Build history of the part. All positions in model axes, mm. A direction names the side the tool comes from. Round coordinates to 2 decimals unless told otherwise and drop trailing zeros. Write each loop counter-clockwise with the first axis right and the second up, starting at its lowest first coordinate (ties: lowest second). Pieces come first, ordered by that corner, then holes. Notation, with made-up numbers: (-16.5, 47.5) - (-7.5, 47.5) arc R19 cw to (-7.5, 70.5) - close; hole circle Ø7 at (-11.75, 17.5). An arc over 180 degrees is marked (long way). One line per question, with ' | ' between items.
from build123d import *

# Parameters (mm, degrees)
SKETCH2_W           = 1.5
SKETCH2_H           = 37.57
SKETCH2_H_2         = 1.5
SKETCH2_W_2         = 39.569
BOSS_EXTRUDE1_DEPTH = 40
SKETCH3_R           = 1.65
CUT_EXTRUDE1_DEPTH  = 40
SKETCH4_R           = 10.5
SKETCH4_R_2         = 1.65
CUT_EXTRUDE2_DEPTH  = 40
FILLET1_R           = 1


with BuildPart() as part:
    # Sketch2 → Boss-Extrude1 (new body)
    with BuildSketch(Plane(origin=(0, 0, 0), x_dir=(0, 0, -1), z_dir=(1, 0, 0))):
        with Locations((-36.139408466, 17.750517241)):
            Rectangle(SKETCH2_W, SKETCH2_H)
        with Locations((-36.139408466, -1.784482759)):
            Rectangle(SKETCH2_W, SKETCH2_H_2)
        with Locations((-15.604908466, -1.784482759)):
            Rectangle(SKETCH2_W_2, SKETCH2_H_2)
    extrude(amount=BOSS_EXTRUDE1_DEPTH)

    # Sketch3 → Cut-Extrude1 (cut)
    with BuildSketch(Plane(origin=(0, -1.034482759, 0), x_dir=(1, 0, 0), z_dir=(0, 1, 0))):
        with Locations(Location((4.5, -30.820408466, 0), (0, 0, 270))):
            Circle(SKETCH3_R)
        with Locations(Location((4.5, -20.820408466, 0), (0, 0, 270))):
            Circle(SKETCH3_R)
        with Locations(Location((4.5, -10.820408466, 0), (0, 0, 270))):
            Circle(SKETCH3_R)
        with Locations(Location((4.5, -0.820408466, 0), (0, 0, 270))):
            Circle(SKETCH3_R)
        with Locations(Location((35.5, -30.820408466, 0), (0, 0, 270))):
            Circle(SKETCH3_R)
        with Locations(Location((35.5, -20.820408466, 0), (0, 0, 270))):
            Circle(SKETCH3_R)
        with Locations(Location((35.5, -10.820408466, 0), (0, 0, 270))):
            Circle(SKETCH3_R)
        with Locations(Location((35.5, -0.820408466, 0), (0, 0, 270))):
            Circle(SKETCH3_R)
    extrude(amount=-CUT_EXTRUDE1_DEPTH, mode=Mode.SUBTRACT)

    # Sketch4 → Cut-Extrude2 (cut)
    with BuildSketch(Plane(origin=(0, 0, 35.389408466), x_dir=(-1, 0, 0), z_dir=(0, 0, -1))):
        with Locations(Location((-20, 16.535517241, 0), (0, 0, 90))):
            Circle(SKETCH4_R)
        with Locations(Location((-11.070998723, 25.983952889, 0), (0, 0, 90))):
            Circle(SKETCH4_R_2)
        with Locations(Location((-10.551564352, 7.606515964, 0), (0, 0, 90))):
            Circle(SKETCH4_R_2)
        with Locations(Location((-29.448435648, 25.464518519, 0), (0, 0, 90))):
            Circle(SKETCH4_R_2)
        with Locations(Location((-28.929001277, 7.087081594, 0), (0, 0, 90))):
            Circle(SKETCH4_R_2)
        with BuildLine():
            Line((-40, 36.535517241), (-40, 16.535517241))
            ThreePointArc((-40, 16.535517241), (-34.142135624, 30.677652865), (-20, 36.535517241))
            Line((-20, 36.535517241), (-40, 36.535517241))
        make_face()
        with BuildLine():
            Line((0, 36.535517241), (-20, 36.535517241))
            ThreePointArc((-20, 36.535517241), (-5.857864785, 30.677653274), (0, 16.535518399))
            Line((0, 16.535518399), (0, 36.535517241))
        make_face()
    extrude(amount=-CUT_EXTRUDE2_DEPTH, mode=Mode.SUBTRACT)

    # Fillet1
    fillet1_edges = [part.edges().sort_by_distance(p)[0] for p in [
        (40, -1.784482759, -4.179591534),
        (0, -1.784482759, -4.179591534),
    ]]
    fillet(fillet1_edges, radius=FILLET1_R)


solid = part.part
Q1. Pull direction X, two halves, no side cores. Call faces 1 (the flat face through (40, -1.4, 22.9)), 2 (the cylindrical face through (4.996, -1.774, 32.394)), 3 (the cylindrical face through (3.868, -1.774, 2.345)), 4 (the flat face through (20, -2, -4.18)): +X half, -X half, draft (parallel to the pull), parting line (faces both ways), or undercut.
Found:
face 1: +X half | face 2: undercut | face 3: undercut | face 4: draft
Q2. Saw through at D-D, the plane y = 2.5. List the corners of the cut face in (x, z).
Found:
outline: (0, 35.39) - (40, 35.39) - (40, 36.89) - (0, 36.89) - close
Q3. Saw through at A-A, the plane y = 15. List the corners of the cut face in (x, z), then the cut area to 3 significant figures.
Found:
outline: (0, 35.39) - (9.61, 35.39) - (9.61, 36.89) - (0, 36.89) - close; (30.39, 35.39) - (40, 35.39) - (40, 36.89) - (30.39, 36.89) - close | area: 28.8 mm^2
Q4. Saw through at B-B, the plane x = 19. List the corners of the cut face in (y, z), then the cut area to 3 significant figures.
Found:
outline: (-2.53, -4.18) - (-1.03, -4.18) - (-1.03, 35.39) - (6.08, 35.39) - (6.08, 36.89) - (-2.53, 36.89) - close; (26.99, 35.39) - (36.51, 35.39) - (36.51, 36.89) - (26.99, 36.89) - close | area: 86.6 mm^2
Q5. Drill centre lines: L1, parallel to Z at x = 35, y = -2; L2, parallel to Z at x = 5.5, y = 1.5; L3, parallel to Y at x = 11, z = 8. Where is each one in solid material? Low to high. Write a range as from..to.
Found:
L1: -4.18..-0.75, 2.39..9.25, 12.39..19.25, 22.39..29.25, 32.39..36.89 | L2: 35.39..36.89 | L3: -2.53..-1.03
Q6. Saw through at C-C, the plane x = 4.5. List the corners of the cut face in (y, z), then the cut area to 3 significant figures.
Found:
outline: (-2.53, -4.18) - (-1.03, -4.18) - (-1.03, -0.83) - (-2.53, -0.83) - close; (-2.53, 2.47) - (-1.03, 2.47) - (-1.03, 9.17) - (-2.53, 9.17) - close; (-2.53, 12.47) - (-1.03, 12.47) - (-1.03, 19.17) - (-2.53, 19.17) - close; (-2.53, 22.47) - (-1.03, 22.47) - (-1.03, 29.17) - (-2.53, 29.17) - close; (-2.53, 32.47) - (-1.03, 32.47) - (-1.03, 35.39) - (29.17, 35.39) - (29.17, 36.89) - (-2.53, 36.89) - close | area: 87.1 mm^2
Q7. Drop flat-ended pins along their axis: pin 1 (3 mm diameter, centred on x = 4.5, z = 20.82, fed in from -Y); pin 2 (5.5 mm diameter, centred on x = 29.45, y = 25.46, fed in from -Z); pin 3 (3 mm diameter, centred on x = 21.5, z = 8.5, fed in from +Y). Give the stop position or say it passes through.
Found:
pin 1: through | pin 2: z = 35.39 | pin 3: y = -1.03
Q8. Which spindle directions (+Z, -Z, +X, -X, +Y, -Y) get a long thin tool onto all of the face, cutting with end or side? Do faces 5 (the flat face through (0, -1.4, 22.9)), 6 (the flat face through (20, -1.034, 16)). Say none if no direction does.
Found:
face 5: +Z, -Z, -X, +Y, -Y | face 6: -Z, +X, -X, +Y
